```python
from build123d import *

# Parameters (mm, degrees)
F2_W     = 205
F2_H     = 125
F3_DEPTH = 25
F4_T     = -5
F5_SIZE  = 5
F6_R     = 5
F7_R     = 2.5
F8_R     = 3.3


with BuildPart() as f3:
    # F2 (on Top) → F3 (new body)
    with BuildSketch(Plane.XY):
        Rectangle(F2_W, F2_H)
    extrude(amount=F3_DEPTH)

    # F4
    f4_openings = [f3.faces().sort_by_distance(p)[0] for p in [
        (0, 0, 25),
    ]]
    offset(amount=F4_T, openings=f4_openings)

    # F5
    f5_edges = [f3.edges().sort_by_distance(p)[0] for p in [
        (0, 62.5, 0),
        (-102.5, 0, 0),
        (0, -62.5, 0),
        (102.5, 0, 0),
    ]]
    chamfer(f5_edges, length=F5_SIZE)

    # F6
    f6_edges = [f3.edges().sort_by_distance(p)[0] for p in [
        (100, -60, 2.5),
        (-100, 60, 2.5),
        (-100, -60, 2.5),
        (100, 60, 2.5),
    ]]
    fillet(f6_edges, radius=F6_R)

    # F7
    f7_edges = [f3.edges().sort_by_distance(p)[0] for p in [
        (-97.5, -57.5, 15),
        (-97.5, 57.5, 15),
        (97.5, 57.5, 15),
        (97.5, -57.5, 15),
        (0, -57.5, 5),
        (97.5, 0, 5),
        (0, 57.5, 5),
        (-97.5, 0, 5),
    ]]
    fillet(f7_edges, radius=F7_R)

    # F8
    f8_edges = [f3.edges().sort_by_distance(p)[0] for p in [
        (102.5, 62.5, 15.473672),
        (102.5, -62.5, 15.473672),
        (-102.5, -62.5, 15.473672),
        (-102.5, 62.5, 15.473672),
    ]]
    fillet(f8_edges, radius=F8_R)


solid = f3.part
```
Check sheet for the modelled part. Datum: model origin and axes. Units: mm. A direction names the side the tool comes from. Coordinates: 2 decimals unless noted, no trailing zeros. Order: outer loops, then holes, each group sorted by start corner. A loop starts at its lowest first (then second) coordinate and runs counter-clockwise, first axis right, second up. Notation, with made-up numbers: M -29,-36 L 8,-36 A15 cw 8,-10 Z; hole C 27,-16 d3. An arc over 180 degrees is marked long. Write each question's results on one line, items separated by ' | '. Start each with the question number.
1. Access from +Z, -Z, +X, -X, +Y, -Y to the whole of each face (thin tool, end or side, straight path). Record for faces 1 (the face through (-1, -57.5, 16)), 2 (the face through (-98.8, -58.7, 2.2)).
2. Mould release check, pull along Y, two halves, no side actions. Record for faces 3 (the face through (100, -0.8, 2.5)), 4 (the face through (-1, 57.5, 16)), 5 (the face through (-1.4, -60, 2.5)): +Y half, -Y half, draft (parallel to the pull), parting line (faces both ways), or undercut.
3. Cross-section at C-C on y = -2. Record the cut outline in (x, z).
4. Cross-section at A-A on z = 14.75. Record the cut outline in (x, y), and give its area (3 significant figures).
5. Material ranges on probe 1 along Y at (x, z) = (83.5, 21.25); probe 2 along X at (y, z) = (-51.5, 15.5); probe 3 along Z at (x, y) = (-45, 53), recorded low to high.
6. Cross-section at B-B on x = -55. Record the cut outline in (y, z).
7. Go/stop test with flat-tipped pins: P1, Ø1.5, axis at x = 18, z = 3, coming from the +Y side; P2, Ø3, axis at x = -19.5, y = 26, coming from the +Z side. Record where each tip stops, or that it passes through.
Checks:
1) face 1: +Z | face 2: -Z, -X, -Y
2) face 3: draft | face 4: undercut | face 5: -Y half
3) outline: M -102.5,5 L -97.5,0 L 97.5,0 L 102.5,5 L 102.5,25 L 97.5,25 L 97.5,7.5 A2.5 cw 95,5 L -95,5 A2.5 cw -97.5,7.5 L -97.5,25 L -102.5,25 Z
4) outline: M -102.5,-59.2 A3.3 ccw -99.2,-62.5 L 99.2,-62.5 A3.3 ccw 102.5,-59.2 L 102.5,59.2 A3.3 ccw 99.2,62.5 L -99.2,62.5 A3.3 ccw -102.5,59.2 Z; hole M -97.5,-55 A2.5 ccw -95,-57.5 L 95,-57.5 A2.5 ccw 97.5,-55 L 97.5,55 A2.5 ccw 95,57.5 L -95,57.5 A2.5 ccw -97.5,55 Z | area: 3,200 mm²
5) probe 1: y = -62.5 to -57.5, 57.5 to 62.5 | probe 2: x = -102.5 to -97.5, 97.5 to 102.5 | probe 3: z = 0 to 5
6) outline: M -62.5,5 L -57.5,0 L 57.5,0 L 62.5,5 L 62.5,25 L 57.5,25 L 57.5,7.5 A2.5 cw 55,5 L -55,5 A2.5 cw -57.5,7.5 L -57.5,25 L -62.5,25 Z
7) P1: stops at y = 61.25 | P2: stops at z = 5
